from build123d import *

# Parameters (mm, degrees)
SKETCH_1_R          = 14
SKETCH_2_R          = 14
SKETCH_10_R         = 8.5
SKETCH_5_R          = 8.5
SKETCH_11_R         = 4.9
SKETCH_8_R          = 4.9
SKETCH_9_R          = 3
SKETCH_12_R         = 3
CUT_EXTRUDE_START   = -17
CUT_EXTRUDE_1_DEPTH = 17


with BuildPart() as part:
    # Эскиз1 → По сечениям2 section 0
    with BuildSketch(Plane(origin=(0, 0, 0), x_dir=(1, 0, 0), z_dir=(0, 1, 0))):
        Circle(SKETCH_1_R)
    # Эскиз2 → По сечениям2 section 1
    with BuildSketch(Plane(origin=(0, 87.2, 0), x_dir=(1, 0, 0), z_dir=(0, 1, 0))):
        Circle(SKETCH_2_R)
    loft()

    # Эскиз10 → По сечениям3 section 0
    with BuildSketch(Plane(origin=(0, 87.2, 0), x_dir=(1, 0, 0), z_dir=(0, 1, 0))):
        Circle(SKETCH_10_R)
    # Эскиз5 → По сечениям3 section 1
    with BuildSketch(Plane(origin=(0, 89.2, 0), x_dir=(1, 0, 0), z_dir=(0, 1, 0))):
        Circle(SKETCH_5_R)
    loft()

    # Эскиз11 → По сечениям4 section 0
    with BuildSketch(Plane(origin=(0, 89.2, 0), x_dir=(1, 0, 0), z_dir=(0, 1, 0))):
        Circle(SKETCH_11_R)
    # Эскиз8 → По сечениям4 section 1
    with BuildSketch(Plane(origin=(0, 90.3, 0), x_dir=(1, 0, 0), z_dir=(0, 1, 0))):
        Circle(SKETCH_8_R)
    loft()

    # Эскиз9 → По сечениям5 section 0
    with BuildSketch(Plane(origin=(0, 107.3, 0), x_dir=(1, 0, 0), z_dir=(0, 1, 0))):
        Circle(SKETCH_9_R)
    # Эскиз12 → По сечениям5 section 1
    with BuildSketch(Plane(origin=(0, 90.3, 0), x_dir=(1, 0, 0), z_dir=(0, 1, 0))):
        Circle(SKETCH_12_R)
    loft()

    # Эскиз13 → Вырез-Вытянуть1 (cut)
    with BuildSketch(Plane(origin=(0, 107.3, 0), x_dir=(1, 0, 0), z_dir=(0, 1, 0)).offset(CUT_EXTRUDE_START)):
        with BuildLine():
            Line((2.4, 1.8), (2.4, -1.8))
            ThreePointArc((2.4, -1.8), (2.846049894, -0.948683298), (3, 0))
            ThreePointArc((3, 0), (2.846049894, 0.948683298), (2.4, 1.8))
        make_face()
    extrude(amount=CUT_EXTRUDE_1_DEPTH, mode=Mode.SUBTRACT)


solid = part.part
Geometry: final body of the model. Coordinates: model frame, mm. A direction names the side the tool comes from. Give positions to 0.01 mm unless a question says otherwise; leave off trailing zeros. Loops run counter-clockwise (first coordinate to the right, second up) from the corner with the lowest first, then second, coordinate; pieces in that order, holes last. Notation, with made-up numbers: M -0.75,20 L 30.25,20 A18 ccw 30.25,48 Z; hole C 72.25,54 d9. An arc over 180 degrees is marked long. Put each result on its own line as item: value. Start each with the question number.
1) Access query for faces 1 (the flat face through (4, 89.2, 4)), 2 (the flat face through (2.4, 99, 0)), 3 (the cylindrical face through (12.932, 44.21, 5.362)). Directions: +Z, -Z, +X, -X, +Y, -Y. A direction counts if a zero-diameter tool reaches every point of the face in a straight line with its end or side. Return the directions, or none.
2) Ray query, line 1 along Y through (x, z) = (-4.5, -9); line 2 along Z through (x, y) = (0.25, 9.5); line 3 along Y through (x, z) = (-0.5, 8). Return the intervals inside material, ascending.
3) Contact query for flat-ended pins moving along their axis: pin 1 (8.5 mm diameter, centred on x = 1, z = 3, fed in from +Y); pin 2 (3 mm diameter, centred on x = 7, y = 45, fed in from -Z); pin 3 (6 mm diameter, centred on x = 0, y = 92, fed in from -Z); pin 4 (1.1 mm diameter, centred on y = 96.5, z = 0.5, fed in from +X). Output: stop coordinate, or through.
4) Cut plane C-C (y = 98). Output: boundary loops of the cut face in (x, z).
5) Cut plane B-B (z = 6). Output: boundary loops of the cut face in (x, y), then the cut area to 3 significant figures.
6) Cut plane A-A (x = 0). Output: boundary loops of the cut face in (y, z).
7) Cut plane D-D (x = -6.75). Output: boundary loops of the cut face in (y, z).
Verdict:
1. face 1: +Y
1. face 2: +Z, -Z, +X, +Y
1. face 3: +Y, -Y
2. line 1: 0 to 87.2
2. line 2: -14 to 14
2. line 3: 0 to 89.2
3. pin 1: y = 107.3
3. pin 2: z = -12.87
3. pin 3: z = -8.5
3. pin 4: x = 2.4
4. outline: M 2.4,-1.8 L 2.4,1.8 A3 ccw long Z
5. outline: M -12.65,0 L 12.65,0 L 12.65,87.2 L 6.02,87.2 L 6.02,89.2 L -6.02,89.2 L -6.02,87.2 L -12.65,87.2 Z
5. area: 2,230 mm2
6. outline: M 0,-14 L 87.2,-14 L 87.2,-8.5 L 89.2,-8.5 L 89.2,-4.9 L 90.3,-4.9 L 90.3,-3 L 107.3,-3 L 107.3,3 L 90.3,3 L 90.3,4.9 L 89.2,4.9 L 89.2,8.5 L 87.2,8.5 L 87.2,14 L 0,14 Z
7. outline: M 0,-12.27 L 87.2,-12.27 L 87.2,-5.17 L 89.2,-5.17 L 89.2,5.17 L 87.2,5.17 L 87.2,12.27 L 0,12.27 Z
